from build123d import *

# Parameters (mm, degrees)
BOSS_EXTRU_1_DEPTH      = 3
CONG_1_R                = 3
ESQUISSE2_R             = 1.75
ENL_V_MAT_EXTRU_1_DEPTH = 33.826209041


with BuildPart() as part:
    # Esquisse1 → Boss.-Extru.1 (new, symmetric)
    with BuildSketch(Plane.XY):
        with BuildLine():
            Line((-26.6, 0), (-19, 0))
            ThreePointArc((-19, 0), (0, 19), (19, 0))
            Line((19, 0), (26.6, 0))
            Line((26.6, 0), (26.6, 0.6))
            Line((26.6, 0.6), (19.590814174, 0.6))
            ThreePointArc((19.590814174, 0.6), (0, 19.6), (-19.590814174, 0.6))
            Line((-19.590814174, 0.6), (-26.6, 0.6))
            Line((-26.6, 0.6), (-26.6, 0))
        make_face()
    extrude(amount=BOSS_EXTRU_1_DEPTH, both=True)

    # Congé1
    cong_1_edges = [part.edges().sort_by_distance(p)[0] for p in [
        (-26.6, 0.3, -3),
        (-26.6, 0.3, 3),
        (26.6, 0.3, -3),
        (26.6, 0.3, 3),
    ]]
    fillet(cong_1_edges, radius=CONG_1_R - 0.0001)  # a hair under: the kernel refuses the full size

    # Esquisse2 → Enlèv. mat.-Extru.1 (cut, through all)
    with BuildSketch(Plane(origin=(0, 0.6, 0), x_dir=(1, 0, 0), z_dir=(0, 1, 0))):
        with Locations(Location((-23.5, 0, 0), (0, 0, 180))):
            Circle(ESQUISSE2_R)
        with Locations(Location((23.5, 0, 0), (0, 0, 180))):
            Circle(ESQUISSE2_R)
    extrude(amount=-ENL_V_MAT_EXTRU_1_DEPTH, mode=Mode.SUBTRACT)


solid = part.part
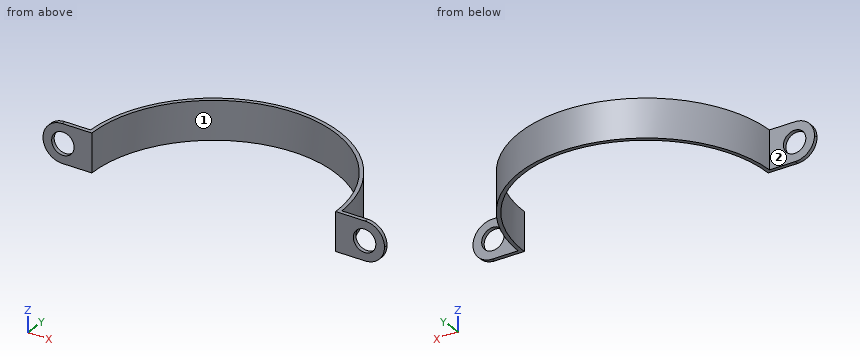
CAD build for the part. Positions are in the model's coordinates, mm. Face numbers are marked on the shaded views. A direction names the side the tool comes from. Give positions to 0.01 mm unless a question says otherwise; leave off trailing zeros. Loops run counter-clockwise (first coordinate to the right, second up) from the corner with the lowest first, then second, coordinate; pieces in that order, holes last. Notation, with made-up numbers: M -37.75,24 L -5.75,24 A25 cw -5.75,41 Z; hole C 0.5,-23 d1. An arc over 180 degrees is marked long. One line per question, with ' | ' between items. Start each with the question number.
1. Flat gauge pins, fed straight in: pin 1 (1 mm diameter, centred on y = 8.5, z = 1, fed in from -X); pin 2 (3 mm diameter, centred on y = 5.5, z = -1, fed in from +X); pin 3 (3 mm diameter, centred on x = -23.5, z = 0, fed in from -Y); pin 4 (3 mm diameter, centred on x = 22, z = -1, fed in from +Y). Where does each tip first touch, or does it go through?
2. Probe L1, parallel to Z at x = -23.5, y = 0.3; L2, parallel to X at y = 3.5, z = -2; L3, parallel to X at y = 2.25, z = 0.5. List the from-to ranges inside material, lowest first. Write a range as from..to.
3. Saw through at A-A on y = 14.25. Give the cut face in (x, z).
4. Saw through at D-D on y = 6. Give the cut face in (x, z), plus the area to 3 significant figures.
5. Saw through at C-C on x = 0. Give the cut face in (y, z).
6. Saw through at B-B on z = 2.25. Give the cut face in (x, y), plus the area to 3 significant figures.
7. 3-axis set-ups, long thin cutter, end or side, ignore diameter. For the marked faces 1 and 2: which of +Z, -Z, +X, -X, +Y, -Y reach the whole face in a straight line?
Result sheet:
1) pin 1: stops at x = -17.89 | pin 2: stops at x = 19.19 | pin 3: passes through | pin 4: stops at y = 0.6
2) L1: z = -3..-1.75, 1.75..3 | L2: x = -19.28..-18.67, 18.67..19.28 | L3: x = -19.47..-18.87, 18.87..19.47
3) outline: M -13.46,-3 L -12.57,-3 L -12.57,3 L -13.46,3 Z; M 12.57,-3 L 13.46,-3 L 13.46,3 L 12.57,3 Z
4) outline: M -18.66,-3 L -18.03,-3 L -18.03,3 L -18.66,3 Z; M 18.03,-3 L 18.66,-3 L 18.66,3 L 18.03,3 Z | area: 7.58 mm^2
5) outline: M 19,-3 L 19.6,-3 L 19.6,3 L 19,3 Z
6) outline: M -25.58,0 L -19,0 A19 cw 19,0 L 25.58,0 L 25.58,0.6 L 19.59,0.6 A19.6 ccw -19.59,0.6 L -25.58,0.6 Z | area: 43.6 mm^2
7) face 1: +Z, -Z, -Y | face 2: +Z, -Z, -X, +Y
